Verification items for the finished model (mm, model axes). Face numbers are marked on the shaded views. Round coordinates to 2 decimals unless told otherwise and drop trailing zeros. Write each loop counter-clockwise with the first axis right and the second up, starting at its lowest first coordinate (ties: lowest second). Pieces come first, ordered by that corner, then holes. Notation, with made-up numbers: (-4.5, 74) - (10.5, 74) arc R28 ccw to (10.5, 106) - close; hole circle Ø5 at (61.25, -17.75). An arc over 180 degrees is marked (long way). Answer as a JSON object with one key per item and string values.
```python
from build123d import *

# Parameters (mm, degrees)
SKETCH1_R                       = 76.2
BOSS_EXTRUDE1_DEPTH             = 3.81
BOSS_EXTRUDE3_DEPTH             = 3.81
SKETCH5_R                       = 6.35
CUT_EXTRUDE1_DEPTH              = 4.81
BOSS_EXTRUDE4_START             = -3.81
BOSS_EXTRUDE4_DEPTH             = 16.51
SKETCH9_R                       = 3.174999999
CUT_EXTRUDE4_DEPTH              = 3.81
SKETCH11_R                      = 31.75
SKETCH11_R_2                    = 25.4
BOSS_EXTRUDE5_DEPTH             = 3.81
SKETCH12_R                      = 25.4
CUT_EXTRUDE5_DEPTH              = 3.81
SKETCH13_R                      = 20.52955
SKETCH13_R_2                    = 2.3622
BOSS_EXTRUDE7_DEPTH             = 3.81
SKETCH14_R                      = 2.3622
CUT_EXTRUDE6_DEPTH              = 3.81
SKETCH15_R                      = 3.175
CUT_EXTRUDE7_DEPTH              = 3.81
TAP_DRILL_FOR_1_4_20_TAP1_D     = 5.1054
TAP_DRILL_FOR_1_4_20_TAP1_DEPTH = 3.087343788
CIRPATTERN1_COUNT               = 4
SKETCH22_R                      = 2.54
CUT_EXTRUDE8_DEPTH              = 17.78


with BuildPart() as part:
    # Sketch1 → Boss-Extrude1 (new body)
    with BuildSketch(Plane(origin=(0, 0, 0), x_dir=(1, 0, 0), z_dir=(0, 1, 0))):
        Circle(SKETCH1_R)
    extrude(amount=BOSS_EXTRUDE1_DEPTH)

    # Sketch3 → Boss-Extrude3 (add)
    with BuildSketch(Plane(origin=(0, 0, 0), x_dir=(-1, 0, 0), z_dir=(0, -1, 0))):
        with BuildLine():
            Line((9.525, -9.525), (148.920700374, -9.525))
            ThreePointArc((148.920700374, -9.525), (149.225, 0), (148.920700374, 9.525))
            Line((148.920700374, 9.525), (9.525, 9.525))
            Line((9.525, 9.525), (9.525, 148.920700374))
            ThreePointArc((9.525, 148.920700374), (0, 149.225), (-9.525, 148.920700374))
            Line((-9.525, 148.920700374), (-9.525, 9.525))
            Line((-9.525, 9.525), (-148.920700374, 9.525))
            ThreePointArc((-148.920700374, 9.525), (-149.225, 0), (-148.920700374, -9.525))
            Line((-148.920700374, -9.525), (-9.525, -9.525))
            Line((-9.525, -9.525), (-9.525, -148.920700374))
            ThreePointArc((-9.525, -148.920700374), (0, -149.225), (9.525, -148.920700374))
            Line((9.525, -148.920700374), (9.525, -9.525))
        make_face()
    extrude(amount=-BOSS_EXTRUDE3_DEPTH)

    # Sketch5 → Cut-Extrude1 (cut, through all)
    with BuildSketch(Plane(origin=(0, 3.81, 0), x_dir=(1, 0, 0), z_dir=(0, 1, 0))):
        Circle(SKETCH5_R)
    extrude(amount=-CUT_EXTRUDE1_DEPTH, mode=Mode.SUBTRACT)

    # Sketch7 → Boss-Extrude4 (add)
    with BuildSketch(Plane(origin=(0, 3.81, 0), x_dir=(1, 0, 0), z_dir=(0, 1, 0)).offset(BOSS_EXTRUDE4_START)):
        with BuildLine():
            Line((18.739703318, 148.043656212), (18.739703318, 146.138656212))
            Line((18.739703318, 146.138656212), (-18.739703318, 146.138656212))
            Line((-18.739703318, 146.138656212), (-18.739703318, 148.043656212))
            ThreePointArc((-18.739703318, 148.043656212), (0, 149.225), (18.739703318, 148.043656212))
        make_face()
    boss_extrude4 = extrude(amount=BOSS_EXTRUDE4_DEPTH)

    # Sketch9 → Cut-Extrude4 (cut)
    with BuildSketch(Plane.XZ):
        with Locations((-56.514999999, -23.8125)):
            Circle(SKETCH9_R)
        with Locations((-15.874999999, -23.8125)):
            Circle(SKETCH9_R)
    extrude(amount=-CUT_EXTRUDE4_DEPTH, mode=Mode.SUBTRACT)

    # Sketch11 → Boss-Extrude5 (add)
    with BuildSketch(Plane(origin=(0, 3.81, 0), x_dir=(1, 0, 0), z_dir=(0, 1, 0))):
        with Locations((41.275, -41.275)):
            Circle(SKETCH11_R)
        with Locations((41.275, -41.275)):
            Circle(SKETCH11_R_2, mode=Mode.SUBTRACT)
    extrude(amount=-BOSS_EXTRUDE5_DEPTH)

    # Sketch12 → Cut-Extrude5 (cut)
    with BuildSketch(Plane(origin=(0, 3.81, 0), x_dir=(1, 0, 0), z_dir=(0, 1, 0))):
        with Locations((41.275, -41.275)):
            Circle(SKETCH12_R)
    extrude(amount=-CUT_EXTRUDE5_DEPTH, mode=Mode.SUBTRACT)

    # Sketch13 → Boss-Extrude7 (add)
    with BuildSketch(Plane(origin=(0, 3.81, 0), x_dir=(1, 0, 0), z_dir=(0, 1, 0))):
        with Locations((-41.16870274, -55.03340443)):
            Circle(SKETCH13_R)
        with Locations((-41.17109409, -70.730891948)):
            Circle(SKETCH13_R_2, mode=Mode.SUBTRACT)
        with Locations((-41.166311391, -39.335916913)):
            Circle(SKETCH13_R_2, mode=Mode.SUBTRACT)
    extrude(amount=-BOSS_EXTRUDE7_DEPTH)

    # Sketch14 → Cut-Extrude6 (cut)
    with BuildSketch(Plane(origin=(0, 3.81, 0), x_dir=(1, 0, 0), z_dir=(0, 1, 0))):
        with Locations((-41.166311391, -39.335916913)):
            Circle(SKETCH14_R)
    extrude(amount=-CUT_EXTRUDE6_DEPTH, mode=Mode.SUBTRACT)

    # Sketch15 → Cut-Extrude7 (cut)
    with BuildSketch(Plane(origin=(0, 3.81, 0), x_dir=(1, 0, 0), z_dir=(0, 1, 0))):
        with Locations((16.720717023, -16.720717023)):
            Circle(SKETCH15_R)
        with Locations((65.829282977, -16.720717023)):
            Circle(SKETCH15_R)
        with Locations((16.720717023, -65.829282977)):
            Circle(SKETCH15_R)
    extrude(amount=-CUT_EXTRUDE7_DEPTH, mode=Mode.SUBTRACT)

    # Tap Drill for 1/4-20 Tap1
    with Locations(Plane(origin=(0, 0, -149.225), x_dir=(-1, 0, 0), z_dir=(0, 0, -1))):
        with Locations((0, 8.255)):
            tap_drill_for_1_4_20_tap1 = Hole(TAP_DRILL_FOR_1_4_20_TAP1_D / 2, depth=TAP_DRILL_FOR_1_4_20_TAP1_DEPTH)

    # CirPattern1: Boss-Extrude4, Tap Drill for 1/4-20 Tap1 ×4 about axis
    cirpattern1_axis = Axis((0, 0, 0), (0, 1, 0))
    for i in range(1, CIRPATTERN1_COUNT):
        add(boss_extrude4.rotate(cirpattern1_axis, i * 360 / CIRPATTERN1_COUNT))
        add(tap_drill_for_1_4_20_tap1.rotate(cirpattern1_axis, i * 360 / CIRPATTERN1_COUNT), mode=Mode.SUBTRACT)

    # Sketch22 → Cut-Extrude8 (cut)
    with BuildSketch(Plane(origin=(0, 3.81, 0), x_dir=(1, 0, 0), z_dir=(0, 1, 0))):
        with Locations((9.676222664, 47.327342728)):
            Circle(SKETCH22_R)
        with Locations((-9.629274443, 47.327342728)):
            Circle(SKETCH22_R)
        with Locations((-28.93477155, 47.327342728)):
            Circle(SKETCH22_R)
    extrude(amount=-CUT_EXTRUDE8_DEPTH, mode=Mode.SUBTRACT)


solid = part.part
```
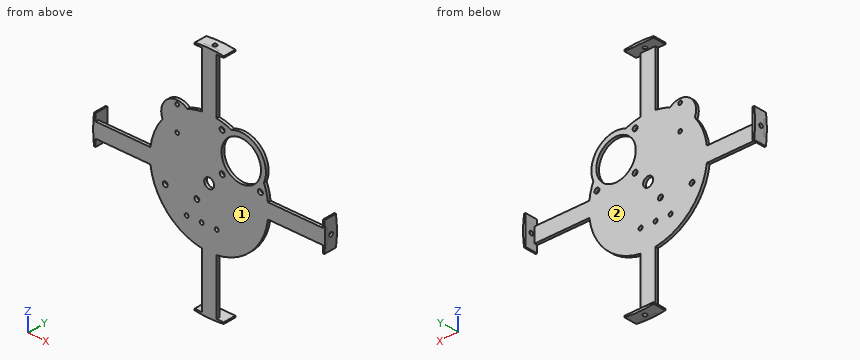
Q1. Section check A-A, the plane z = -87. Record the cut outline in (x, y) (3 decimals), then the cut area to 3 significant figures.
Geometry check:
{"outline": "(-9.525, 0) - (9.525, 0) - (9.525, 3.81) - (-9.525, 3.81) - close", "area": "72.6 mm2"}
Q2. Release check for a two-part mould opening along Z. For the marked faces 1 and 2 record: released by +Z, released by -Z, zero draft, split by the parting line, or undercut.
Geometry check:
{"face 1": "zero draft", "face 2": "undercut"}
Q3. Gauge pin test, flat ends, axial feed: P1, Ø4, axis at x = -127, y = 1, coming from the +Z side (3 decimals); P2, Ø6, axis at x = -41.17, z = 70.73, coming from the +Y side; P3, Ø3, axis at x = -39, z = 20.5, coming from the -Y side; P4, Ø8.5, axis at y = 7.5, z = 8, coming from the -X side. Record the tip position at first contact, or that the pin passes through.
Geometry check:
{"P1": "stops at z = 9.525", "P2": "stops at y = 3.81", "P3": "stops at y = 0", "P4": "stops at x = -149.18"}
Q4. Section check B-B, the plane z = -55.5. Record the cut outline in (x, y), then the cut area to 3 significant figures.
Geometry check:
{"outline": "(-52.21, 0) - (52.21, 0) - (52.21, 3.81) - (-52.21, 3.81) - close", "area": "398 mm2"}
Q5. Material ranges on line 1 along Y through (x, z) = (-147.9, 0); line 2 along Z through (x, y) = (0, 1.9) (3 decimals); line 3 along Z through (x, y) = (3.5, 3.5), recorded low to high. Write a range as [from, to].
Geometry check:
{"line 1": "y = [0, 5.7], [10.81, 16.51]", "line 2": "z = [-149.225, -6.35], [6.35, 149.225]", "line 3": "z = [-149.18, -5.3], [5.3, 149.18]"}
